Design review of the part built by this model. Coordinates are the model's own, in mm. Face numbers are marked on the shaded views. A direction names the side the tool comes from. Give positions to 0.01 mm unless a question says otherwise; leave off trailing zeros. Write each loop counter-clockwise with the first axis right and the second up, starting at its lowest first coordinate (ties: lowest second). Pieces come first, ordered by that corner, then holes. Notation, with made-up numbers: (73.5, 42.25) -> (124.5, 42.25) arc R10 ccw to (124.5, 46.25) -> close; hole circle Ø7 at (-8, 0.5). An arc over 180 degrees is marked (long way). Use CSV: the item, a comma, the result in double quotes.
```python
from build123d import *

# Parameters (mm, degrees)
F1_DEPTH = 6.35
F2_R     = 2.921
F3_DEPTH = 6.35


with BuildPart() as f1:
    # F0 (on Right) → F1 (new body)
    with BuildSketch(Plane.YZ):
        Polygon((-16.51, 0), (0, 0), (0, 35.56), (-8.89, 35.56), (-8.89, 7.62), (-16.51, 7.62), align=None)
    extrude(amount=F1_DEPTH)

    # F2 (on face) → F3 (join)
    with BuildSketch(Plane.YZ.offset(6.35)):
        with Locations((-4.445, 30.48)):
            Circle(F2_R)
    extrude(amount=F3_DEPTH)


solid = f1.part
```
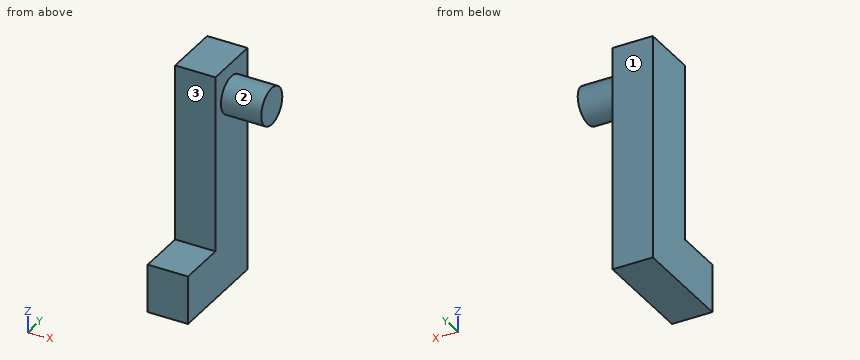
(1) Clearance check with a flat-ended pin moving along its axis: pin 1 (1.9 mm diameter, centred on x = 3.5, z = 19.5, fed in from -Y). State where the tip first meets the part, or that it passes through.
Established:
pin 1,"stops at y = -8.89"
(2) Take a section at D-D (x = 8.75). Write out the cut boundary in (y, z) (3 decimals), then the cut area to 3 significant figures.
Established:
outline,"circle Ø5.842 at (-4.445, 30.48)"
area,"26.8 mm2"
(3) Take a section at A-A (z = 30.48). Write out the cut boundary in (x, y).
Established:
outline,"(0, -8.89) -> (6.35, -8.89) -> (6.35, -7.37) -> (12.7, -7.37) -> (12.7, -1.52) -> (6.35, -1.52) -> (6.35, 0) -> (0, 0) -> close"
(4) Take a section at B-B (x = 3.75). Write out the cut boundary in (y, z).
Established:
outline,"(-16.51, 0) -> (0, 0) -> (0, 35.56) -> (-8.89, 35.56) -> (-8.89, 7.62) -> (-16.51, 7.62) -> close"
(5) For line 1 along Y through (x, z) = (4.5, 33.5); line 2 along X through (y, z) = (-8.5, 15); line 3 along Z through (x, y) = (4.25, -12.75), list the stretches that pass through material, from the lowest coordinate up. Write a range as [from, to].
Established:
line 1,"y = [-8.89, 0]"
line 2,"x = [0, 6.35]"
line 3,"z = [0, 7.62]"
(6) Tool access review of the marked faces 1, 2 and 3: name each direction out of +Z, -Z, +X, -X, +Y, -Y from which nothing blocks a thin tool from reaching the whole face with its end or side.
Established:
face 1,"+Z, -Z, +X, -X, +Y"
face 2,"+X"
face 3,"+Z, +X, -X, -Y"
(7) Take a section at C-C (y = -14.5). Write out the cut boundary in (x, z), then the cut area to 3 significant figures.
Established:
outline,"(0, 0) -> (6.35, 0) -> (6.35, 7.62) -> (0, 7.62) -> close"
area,"48.4 mm2"
